Geometry: final body of the model. Coordinates: model frame, mm. Face numbers are marked on the shaded views. A direction names the side the tool comes from. Give positions to 0.01 mm unless a question says otherwise; leave off trailing zeros. Write each loop counter-clockwise with the first axis right and the second up, starting at its lowest first coordinate (ties: lowest second). Pieces come first, ordered by that corner, then holes.
```python
from build123d import *
from OCP.BRepFilletAPI import BRepFilletAPI_MakeChamfer

# Parameters (mm, degrees)
SKETCH_1_W                          = 12.78
SKETCH_1_H                          = 10.8
EXTRUDE_1_DEPTH                     = 13
FILLET_1_SIZE                       = 1
FILLET_1_SIZE_2                     = 1.5
SKETCH_2_W                          = 2
SKETCH_2_H                          = 3.5
EXTRUDE_2_DEPTH                     = 3.95
SKETCH_3_R                          = 1.5
CUT_EXTRUDE_1_DEPTH                 = 3.95
SKETCH_4_W                          = 0.5
SKETCH_4_H                          = 0.8
EXTRUDE_3_DEPTH                     = 3.5
CHAMFER_1_SIZE                      = 0.5
CHAMFER_1_SIZE2                     = 0.288675135
PATTERN_LINEAR_2_COUNT              = 3
PATTERN_LINEAR_2_PITCH              = 3.81
CHAMFER_1_OF_PATTERN_LINEAR_2_SIZE  = 0.5
CHAMFER_1_OF_PATTERN_LINEAR_2_SIZE2 = 0.288675135


with BuildPart() as part:
    # Эскиз1 → Бобышка-Вытянуть1 (new body)
    with BuildSketch(Plane.XY):
        Rectangle(SKETCH_1_W, SKETCH_1_H)
    extrude(amount=EXTRUDE_1_DEPTH)

    # Скругление1
    # an asymmetric fillet: 1.5, 1 mm, written as the material it takes off along each edge
    with BuildSketch(Plane(origin=(-10.14, -5.4, 13), x_dir=(0, 0, -1), z_dir=(1, 0, 0))) as fillet_1_piece_1:
        with BuildLine():
            Bezier((FILLET_1_SIZE, 0), (0, 0), (0, FILLET_1_SIZE_2), weights=[1, 0.707106781, 1])
            Line((0, FILLET_1_SIZE_2), (0, 0))
            Line((0, 0), (FILLET_1_SIZE, 0))
        make_face()
    extrude(amount=20.28, mode=Mode.SUBTRACT)

    # Эскиз2 → Бобышка-Вытянуть2 (add)
    with BuildSketch(Plane.XY.offset(13)):
        with Locations((3.58, 2.4)):
            Rectangle(SKETCH_2_W, SKETCH_2_H)
    extrude_2 = extrude(amount=EXTRUDE_2_DEPTH)

    # Эскиз3 → Вырез-Вытянуть1 (cut)
    with BuildSketch(Plane.XY.offset(13)):
        with Locations((4.29, -1.686021073)):
            Circle(SKETCH_3_R)
    cut_extrude_1 = extrude(amount=-CUT_EXTRUDE_1_DEPTH, mode=Mode.SUBTRACT)

    # Эскиз4 → Бобышка-Вытянуть3 (add)
    with BuildSketch(Plane(origin=(0, 0, 0), x_dir=(-1, 0, 0), z_dir=(0, 0, -1))):
        with Locations((-5.35, 2.85)):
            Rectangle(SKETCH_4_W, SKETCH_4_H)
        with Locations((-5.35, -2.15)):
            Rectangle(SKETCH_4_W, SKETCH_4_H)
    extrude_3 = extrude(amount=EXTRUDE_3_DEPTH)

    # Фаска1: one chamfer whose edges measure the first distance from different faces: ONE call of the kernel's chamfer builder (chamfer() names one face for all edges)
    chamfer_1_edges_1 = [part.edges().sort_by_distance(p)[0] for p in [
        (5.35, 3.25, -3.5),
    ]]
    chamfer_1_side_1 = [part.faces().sort_by_distance(p)[0] for p in [
        (5.35, 3.25, -1.75),
    ]]
    chamfer_1_edges_2 = [part.edges().sort_by_distance(p)[0] for p in [
        (5.35, 2.45, -3.5),
    ]]
    chamfer_1_side_2 = [part.faces().sort_by_distance(p)[0] for p in [
        (5.35, 2.45, -1.75),
    ]]
    chamfer_1_edges_3 = [part.edges().sort_by_distance(p)[0] for p in [
        (5.35, -2.55, -3.5),
    ]]
    chamfer_1_side_3 = [part.faces().sort_by_distance(p)[0] for p in [
        (5.35, -2.55, -1.75),
    ]]
    chamfer_1_edges_4 = [part.edges().sort_by_distance(p)[0] for p in [
        (5.35, -1.75, -3.5),
    ]]
    chamfer_1_side_4 = [part.faces().sort_by_distance(p)[0] for p in [
        (5.35, -1.75, -1.75),
    ]]
    chamfer_1 = BRepFilletAPI_MakeChamfer(part.part.solid().wrapped)
    for e in chamfer_1_edges_1:
        chamfer_1.Add(CHAMFER_1_SIZE, CHAMFER_1_SIZE2, e.wrapped, chamfer_1_side_1[0].wrapped)  # the first distance lies on this face
    for e in chamfer_1_edges_2:
        chamfer_1.Add(CHAMFER_1_SIZE, CHAMFER_1_SIZE2, e.wrapped, chamfer_1_side_2[0].wrapped)  # the first distance lies on this face
    for e in chamfer_1_edges_3:
        chamfer_1.Add(CHAMFER_1_SIZE, CHAMFER_1_SIZE2, e.wrapped, chamfer_1_side_3[0].wrapped)  # the first distance lies on this face
    for e in chamfer_1_edges_4:
        chamfer_1.Add(CHAMFER_1_SIZE, CHAMFER_1_SIZE2, e.wrapped, chamfer_1_side_4[0].wrapped)  # the first distance lies on this face
    add(Compound.cast(chamfer_1.Shape()), mode=Mode.REPLACE)

    # Линейный массив2: Бобышка-Вытянуть2, Вырез-Вытянуть1, Бобышка-Вытянуть3 ×3
    with Locations(*[(-i * PATTERN_LINEAR_2_PITCH, 0, 0) for i in range(1, PATTERN_LINEAR_2_COUNT)]):
        add(extrude_2)
        add(cut_extrude_1, mode=Mode.SUBTRACT)
        add(extrude_3)

    # Фаска1 of Линейный массив2: one chamfer whose edges measure the first distance from different faces: ONE call of the kernel's chamfer builder (chamfer() names one face for all edges)
    chamfer_1_of_pattern_linear_2_edges_1 = [part.edges().sort_by_distance(p)[0] for p in [
        (1.54, 3.25, -3.5),
    ]]
    chamfer_1_of_pattern_linear_2_side_1 = [part.faces().sort_by_distance(p)[0] for p in [
        (1.54, 3.25, -1.75),
    ]]
    chamfer_1_of_pattern_linear_2_edges_2 = [part.edges().sort_by_distance(p)[0] for p in [
        (1.54, 2.45, -3.5),
    ]]
    chamfer_1_of_pattern_linear_2_side_2 = [part.faces().sort_by_distance(p)[0] for p in [
        (1.54, 2.45, -1.75),
    ]]
    chamfer_1_of_pattern_linear_2_edges_3 = [part.edges().sort_by_distance(p)[0] for p in [
        (1.54, -2.55, -3.5),
    ]]
    chamfer_1_of_pattern_linear_2_side_3 = [part.faces().sort_by_distance(p)[0] for p in [
        (1.54, -2.55, -1.75),
    ]]
    chamfer_1_of_pattern_linear_2_edges_4 = [part.edges().sort_by_distance(p)[0] for p in [
        (1.54, -1.75, -3.5),
    ]]
    chamfer_1_of_pattern_linear_2_side_4 = [part.faces().sort_by_distance(p)[0] for p in [
        (1.54, -1.75, -1.75),
    ]]
    chamfer_1_of_pattern_linear_2_edges_5 = [part.edges().sort_by_distance(p)[0] for p in [
        (-2.27, 3.25, -3.5),
    ]]
    chamfer_1_of_pattern_linear_2_side_5 = [part.faces().sort_by_distance(p)[0] for p in [
        (-2.27, 3.25, -1.75),
    ]]
    chamfer_1_of_pattern_linear_2_edges_6 = [part.edges().sort_by_distance(p)[0] for p in [
        (-2.27, 2.45, -3.5),
    ]]
    chamfer_1_of_pattern_linear_2_side_6 = [part.faces().sort_by_distance(p)[0] for p in [
        (-2.27, 2.45, -1.75),
    ]]
    chamfer_1_of_pattern_linear_2_edges_7 = [part.edges().sort_by_distance(p)[0] for p in [
        (-2.27, -2.55, -3.5),
    ]]
    chamfer_1_of_pattern_linear_2_side_7 = [part.faces().sort_by_distance(p)[0] for p in [
        (-2.27, -2.55, -1.75),
    ]]
    chamfer_1_of_pattern_linear_2_edges_8 = [part.edges().sort_by_distance(p)[0] for p in [
        (-2.27, -1.75, -3.5),
    ]]
    chamfer_1_of_pattern_linear_2_side_8 = [part.faces().sort_by_distance(p)[0] for p in [
        (-2.27, -1.75, -1.75),
    ]]
    chamfer_1_of_pattern_linear_2 = BRepFilletAPI_MakeChamfer(part.part.solid().wrapped)
    for e in chamfer_1_of_pattern_linear_2_edges_1:
        chamfer_1_of_pattern_linear_2.Add(CHAMFER_1_OF_PATTERN_LINEAR_2_SIZE, CHAMFER_1_OF_PATTERN_LINEAR_2_SIZE2, e.wrapped, chamfer_1_of_pattern_linear_2_side_1[0].wrapped)  # the first distance lies on this face
    for e in chamfer_1_of_pattern_linear_2_edges_2:
        chamfer_1_of_pattern_linear_2.Add(CHAMFER_1_OF_PATTERN_LINEAR_2_SIZE, CHAMFER_1_OF_PATTERN_LINEAR_2_SIZE2, e.wrapped, chamfer_1_of_pattern_linear_2_side_2[0].wrapped)  # the first distance lies on this face
    for e in chamfer_1_of_pattern_linear_2_edges_3:
        chamfer_1_of_pattern_linear_2.Add(CHAMFER_1_OF_PATTERN_LINEAR_2_SIZE, CHAMFER_1_OF_PATTERN_LINEAR_2_SIZE2, e.wrapped, chamfer_1_of_pattern_linear_2_side_3[0].wrapped)  # the first distance lies on this face
    for e in chamfer_1_of_pattern_linear_2_edges_4:
        chamfer_1_of_pattern_linear_2.Add(CHAMFER_1_OF_PATTERN_LINEAR_2_SIZE, CHAMFER_1_OF_PATTERN_LINEAR_2_SIZE2, e.wrapped, chamfer_1_of_pattern_linear_2_side_4[0].wrapped)  # the first distance lies on this face
    for e in chamfer_1_of_pattern_linear_2_edges_5:
        chamfer_1_of_pattern_linear_2.Add(CHAMFER_1_OF_PATTERN_LINEAR_2_SIZE, CHAMFER_1_OF_PATTERN_LINEAR_2_SIZE2, e.wrapped, chamfer_1_of_pattern_linear_2_side_5[0].wrapped)  # the first distance lies on this face
    for e in chamfer_1_of_pattern_linear_2_edges_6:
        chamfer_1_of_pattern_linear_2.Add(CHAMFER_1_OF_PATTERN_LINEAR_2_SIZE, CHAMFER_1_OF_PATTERN_LINEAR_2_SIZE2, e.wrapped, chamfer_1_of_pattern_linear_2_side_6[0].wrapped)  # the first distance lies on this face
    for e in chamfer_1_of_pattern_linear_2_edges_7:
        chamfer_1_of_pattern_linear_2.Add(CHAMFER_1_OF_PATTERN_LINEAR_2_SIZE, CHAMFER_1_OF_PATTERN_LINEAR_2_SIZE2, e.wrapped, chamfer_1_of_pattern_linear_2_side_7[0].wrapped)  # the first distance lies on this face
    for e in chamfer_1_of_pattern_linear_2_edges_8:
        chamfer_1_of_pattern_linear_2.Add(CHAMFER_1_OF_PATTERN_LINEAR_2_SIZE, CHAMFER_1_OF_PATTERN_LINEAR_2_SIZE2, e.wrapped, chamfer_1_of_pattern_linear_2_side_8[0].wrapped)  # the first distance lies on this face
    add(Compound.cast(chamfer_1_of_pattern_linear_2.Shape()), mode=Mode.REPLACE)


solid = part.part
```
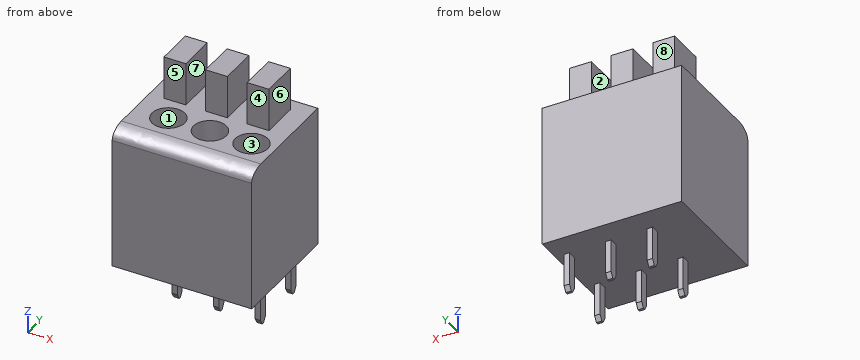
Item 1: Section B-B, the plane y = -3.5. Return the cut outline in (x, z).
Found:
outline: (-6.39, 0) - (6.39, 0) - (6.39, 13) - (-6.39, 13) - close
Item 2: Pull-direction query (Y, two-part tool) for the marked faces 1, 2, 3 and 4; classes: +Y half, -Y half, draft (parallel to the pull), parting line (faces both ways), or undercut.
Found:
face 1: undercut
face 2: draft
face 3: undercut
face 4: -Y half
Item 3: Line query: L1, parallel to X at y = -2, z = -1.25; L2, parallel to X at y = 4, z = 15.5; L3, parallel to Y at x = -3.33, z = 10.9. Output: solid intervals per line, ascending.
Found:
L1: x = -2.52 to -2.02, 1.29 to 1.79, 5.1 to 5.6
L2: x = -5.04 to -3.04, -1.23 to 0.77, 2.58 to 4.58
L3: y = -5.4 to -3.19, -0.19 to 5.4
Item 4: Section A-A, the plane z = 13.5. Return the cut outline in (x, y), plus the area to 3 significant figures.
Found:
outline: (-5.04, 0.65) - (-3.04, 0.65) - (-3.04, 4.15) - (-5.04, 4.15) - close; (-1.23, 0.65) - (0.77, 0.65) - (0.77, 4.15) - (-1.23, 4.15) - close; (2.58, 0.65) - (4.58, 0.65) - (4.58, 4.15) - (2.58, 4.15) - close
area: 21.0 mm2
Item 5: Reachability of the marked faces 5, 6, 7 and 8 from +Z, -Z, +X, -X, +Y, -Y: full face, straight path, thin tool, end or side. Return the list, or none.
Found:
face 5: +Z, +X, -X, -Y
face 6: +Z, +X, +Y, -Y
face 7: +Z, +Y, -Y
face 8: +Z, +X, -X, +Y
Item 6: Pin query (flat end, axial travel): pin 1 Ø0.6 at (y, z) = (-2, -2) entering from +X; pin 2 Ø3.5 at (x, y) = (5, -1.5) entering from +Z; pin 3 Ø1.8 at (y, z) = (1.5, 14.5) entering from +X. Return the tip coordinate at first contact, or that it passes through.
Found:
pin 1: stops at x = 5.6
pin 2: stops at z = 13
pin 3: stops at x = 4.58
